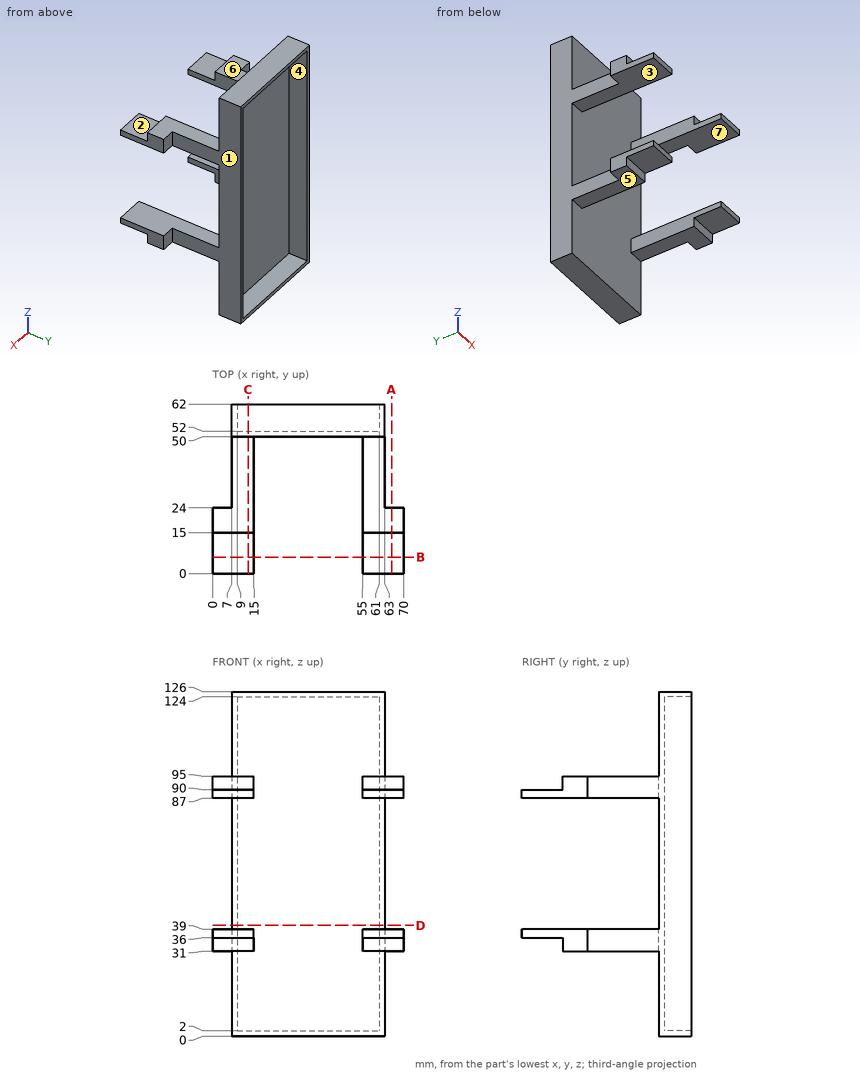
Print and shaded views of the part. All mm, measured from the part's lowest x, y and z. A direction names the side the tool comes from. Round coordinates to 2 decimals unless told otherwise and drop trailing zeros. Write each loop counter-clockwise with the first axis right and the second up, starting at its lowest first coordinate (ties: lowest second). Pieces come first, ordered by that corner, then holes. Notation, with made-up numbers: (0, 9.25) -> (50, 9.25) arc R30 cw to (50, 37.25) -> close; hole circle Ø2 at (62, -28). An arc over 180 degrees is marked (long way). Return JSON: item names as keys, results as strings. Group by question number.
Q1. Saw through at A-A on x = 65.5. Write the cut outline in (y, z).
Q2. Saw through at C-C on x = 13. Write the cut outline in (y, z).
Q3. Saw through at B-B on y = 6. Write the cut outline in (x, z), plus the area to 3 significant figures.
Q4. Mould opens along Z. For the marked faces 1, 2, 3 and 4 say: pulls with the +Z half, pulls with the -Z half, needs draft (parallel to the pull), parting line crosses it, or undercut.
Q5. Pin check, flat tips, straight feed: pin 1 (1 mm diameter, centred on x = 54, z = 94, fed in from +Y); pin 2 (12 mm diameter, centred on x = 59.5, y = 32.5, fed in from +Z); pin 3 (4.5 mm diameter, centred on x = 64, y = 10, fed in from +Z); pin 4 (8 mm diameter, centred on x = 28.5, y = 55, fed in from -Z). Stop position of each tip, or through.
Q6. Which spindle directions (+Z, -Z, +X, -X, +Y, -Y) get a long thin tool onto all of the face, cutting with end or side? Do the marked faces 5, 6 and 7. Say none if no direction does.
Q7. Saw through at D-D on z = 40.5. Write the cut outline in (x, y).
Q8. Probe L1, parallel to X at y = 56, z = 28; L2, parallel to Z at x = 6, y = 13.5; L3, parallel to Y at x = 62, z = 41. List the from-to ranges inside material, lowest first. Write a range as [from, to].
Answer:
{
 "1": {"outline": "(0, 36) -> (15, 36) -> (15, 31) -> (24, 31) -> (24, 39) -> (0, 39) -> close; (0, 87) -> (24, 87) -> (24, 95) -> (15, 95) -> (15, 90) -> (0, 90) -> close"},
 "2": {"outline": "(0, 36) -> (15, 36) -> (15, 31) -> (50, 31) -> (50, 0) -> (62, 0) -> (62, 2) -> (52, 2) -> (52, 124) -> (62, 124) -> (62, 126) -> (50, 126) -> (50, 95) -> (15, 95) -> (15, 90) -> (0, 90) -> (0, 87) -> (50, 87) -> (50, 39) -> (0, 39) -> close"},
 "3": {"outline": "(0, 36) -> (15, 36) -> (15, 39) -> (0, 39) -> close; (0, 87) -> (15, 87) -> (15, 90) -> (0, 90) -> close; (55, 36) -> (70, 36) -> (70, 39) -> (55, 39) -> close; (55, 87) -> (70, 87) -> (70, 90) -> (55, 90) -> close", "area": "180 mm2"},
 "4": {"face 1": "needs draft", "face 2": "pulls with the +Z half", "face 3": "undercut", "face 4": "undercut"},
 "5": {"pin 1": "y = 52", "pin 2": "z = 95", "pin 3": "z = 90", "pin 4": "z = 0"},
 "6": {"face 5": "-Z, +X, -X, -Y", "face 6": "+Z, +X, -X, -Y", "face 7": "+X, -X, -Y"},
 "7": {"outline": "(7, 50) -> (63, 50) -> (63, 62) -> (61, 62) -> (61, 52) -> (9, 52) -> (9, 62) -> (7, 62) -> close"},
 "8": {"L1": "[7, 9], [61, 63]", "L2": "[36, 39], [87, 90]", "L3": "[50, 62]"}
}
